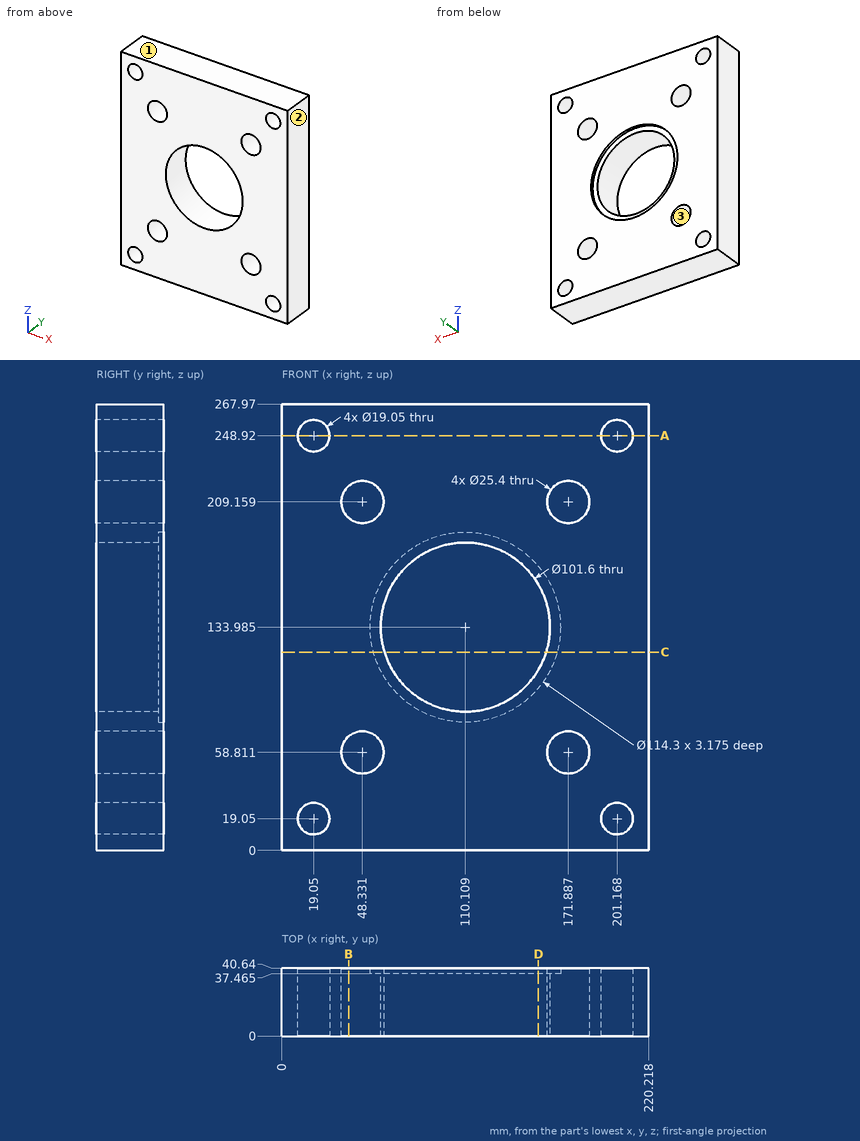
Geometry: see drawing. Coordinates: mm, zero at the bounding-box minimum. Round coordinates to 2 decimals unless told otherwise and drop trailing zeros. Loops run counter-clockwise (first coordinate to the right, second up) from the corner with the lowest first, then second, coordinate; pieces in that order, holes last. Notation, with made-up numbers: (78.25, 56.5) -> (132.25, 56.5) arc R11 cw to (132.25, 75.5) -> close; hole circle Ø2 at (-22.5, 15.25). An arc over 180 degrees is marked (long way). One line per question, with ' | ' between items. Start each with the question number.
1. Section D-D on x = 154. Output: boundary loops of the cut face in (y, z) (1 decimal), and give its area (3 significant figures).
2. Line query: line 1 along Z through (x, y) = (201, 34); line 2 along Z through (x, y) = (110, 7) (1 decimal); line 3 along X through (y, z) = (31, 198.5) (1 decimal). Output: solid intervals per line, ascending. Write a range as [from, to].
3. Section A-A on z = 248.92. Output: boundary loops of the cut face in (x, y) (1 decimal).
4. Mould query, pull axis Z, two halves, no side actions, for the marked faces 1, 2 and 3. Classes: pulls with the +Z half, pulls with the -Z half, needs draft (parallel to the pull), parting line crosses it, or undercut.
5. Section B-B on x = 40. Output: boundary loops of the cut face in (y, z) (1 decimal), and give its area (3 significant figures).
6. Contact query for flat-ended pins moving along their axis: pin 1 (20.5 mm diameter, centred on x = 171.89, z = 58.81, fed in from +Y); pin 2 (22 mm diameter, centred on x = 201.168, z = 248.92, fed in from +Y); pin 3 (6 mm diameter, centred on x = 64.5, z = 105, fed in from +Y) (3 decimals). Output: stop coordinate, or through.
7. Section C-C on z = 119. Output: boundary loops of the cut face in (x, y) (1 decimal).
Returned:
1) outline: (0, 0) -> (40.6, 0) -> (40.6, 97.4) -> (37.5, 97.4) -> (37.5, 108.4) -> (0, 108.4) -> close; (0, 159.6) -> (37.5, 159.6) -> (37.5, 170.6) -> (40.6, 170.6) -> (40.6, 268) -> (0, 268) -> close | area: 8,740 mm2
2) line 1: z = [0, 9.53], [28.57, 239.4], [258.44, 267.97] | line 2: z = [0, 83.2], [184.8, 268] | line 3: x = [0, 41.4], [55.2, 165], [178.8, 220.2]
3) outline: (0, 0) -> (9.5, 0) -> (9.5, 40.6) -> (0, 40.6) -> close; (28.6, 0) -> (191.6, 0) -> (191.6, 40.6) -> (28.6, 40.6) -> close; (210.7, 0) -> (220.2, 0) -> (220.2, 40.6) -> (210.7, 40.6) -> close
4) face 1: pulls with the +Z half | face 2: needs draft | face 3: undercut
5) outline: (0, 0) -> (40.6, 0) -> (40.6, 49.2) -> (0, 49.2) -> close; (0, 68.4) -> (40.6, 68.4) -> (40.6, 199.6) -> (0, 199.6) -> close; (0, 218.7) -> (40.6, 218.7) -> (40.6, 268) -> (0, 268) -> close | area: 9,330 mm2
6) pin 1: passes through | pin 2: stops at y = 40.64 | pin 3: stops at y = 37.465
7) outline: (0, 0) -> (61.6, 0) -> (61.6, 37.5) -> (55, 37.5) -> (55, 40.6) -> (0, 40.6) -> close; (158.6, 0) -> (220.2, 0) -> (220.2, 40.6) -> (165.3, 40.6) -> (165.3, 37.5) -> (158.6, 37.5) -> close
